For this review, use the dimensioned drawing (mm, ordinates from the lowest corner) and the shaded views. Coordinates: 2 decimals unless noted, no trailing zeros. Write each loop counter-clockwise with the first axis right and the second up, starting at its lowest first coordinate (ties: lowest second). Pieces come first, ordered by that corner, then holes. Notation, with made-up numbers: (27.5, 25) - (83.5, 25) arc R24 cw to (83.5, 38) - close; hole circle Ø7 at (-33, -22). An arc over 180 degrees is marked (long way). Answer as a JSON object with one key per item and string values.
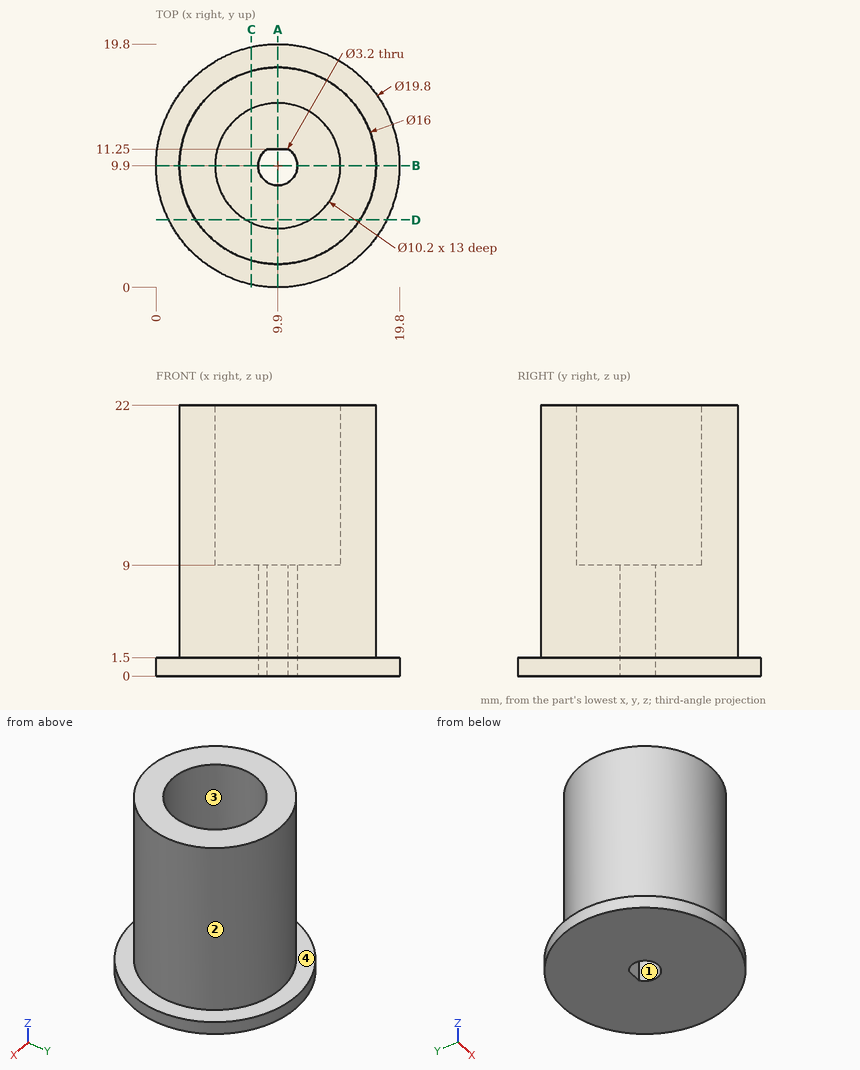
(1) The part is to be moulded in two halves that separate along X. For the marked faces 1, 2, 3 and 4, say which applies: pulls with the +X half, pulls with the -X half, needs draft (parallel to the pull), parting line crosses it, or undercut.
Solved:
{"face 1": "undercut", "face 2": "parting line crosses it", "face 3": "undercut", "face 4": "needs draft"}
(2) Take a section at C-C, the plane x = 7.75. Write out the cut boundary in (y, z).
Solved:
{"outline": "(0.24, 0) - (19.56, 0) - (19.56, 1.5) - (17.61, 1.5) - (17.61, 22) - (14.52, 22) - (14.52, 9) - (5.28, 9) - (5.28, 22) - (2.19, 22) - (2.19, 1.5) - (0.24, 1.5) - close"}
(3) To check wall thickness, follow line 1 (Y direction, x = 9.9, z = 4.25); line 2 (Y direction, x = 9.9, z = 17.25); line 3 (X direction, y = 9.9, z = 5.5). State the ranges of each line that lie inside material, in increasing order. Write a range as from..to.
Solved:
{"line 1": "y = 1.9..8.3, 11.25..17.9", "line 2": "y = 1.9..4.8, 15..17.9", "line 3": "x = 1.9..8.3, 11.5..17.9"}
(4) Take a section at D-D, the plane y = 5.5. Write out the cut boundary in (x, z).
Solved:
{"outline": "(1.03, 0) - (18.77, 0) - (18.77, 1.5) - (16.58, 1.5) - (16.58, 22) - (12.48, 22) - (12.48, 9) - (7.32, 9) - (7.32, 22) - (3.22, 22) - (3.22, 1.5) - (1.03, 1.5) - close"}
(5) Take a section at B-B, the plane y = 9.9. Write out the cut boundary in (x, z), and give its area (3 significant figures).
Solved:
{"outline": "(0, 0) - (8.3, 0) - (8.3, 9) - (4.8, 9) - (4.8, 22) - (1.9, 22) - (1.9, 1.5) - (0, 1.5) - close; (11.5, 0) - (19.8, 0) - (19.8, 1.5) - (17.9, 1.5) - (17.9, 22) - (15, 22) - (15, 9) - (11.5, 9) - close", "area": "196 mm^2"}
(6) Take a section at A-A, the plane x = 9.9. Write out the cut boundary in (y, z), and give its area (3 significant figures).
Solved:
{"outline": "(0, 0) - (8.3, 0) - (8.3, 9) - (4.8, 9) - (4.8, 22) - (1.9, 22) - (1.9, 1.5) - (0, 1.5) - close; (11.25, 0) - (19.8, 0) - (19.8, 1.5) - (17.9, 1.5) - (17.9, 22) - (15, 22) - (15, 9) - (11.25, 9) - close", "area": "199 mm^2"}
(7) For pin 1 (2 mm diameter, centred on x = 14.5, z = 17, fed in from -Y); pin 2 (1 mm diameter, centred on x = 9, z = 14, fed in from +Y); pin 3 (6 mm diameter, centred on y = 11, z = 18.5, fed in from +X), all flat-tipped, find the tip position at first contact; note any pin that passes through.
Solved:
{"pin 1": "stops at y = 2.76", "pin 2": "stops at y = 17.89", "pin 3": "stops at x = 17.9"}
